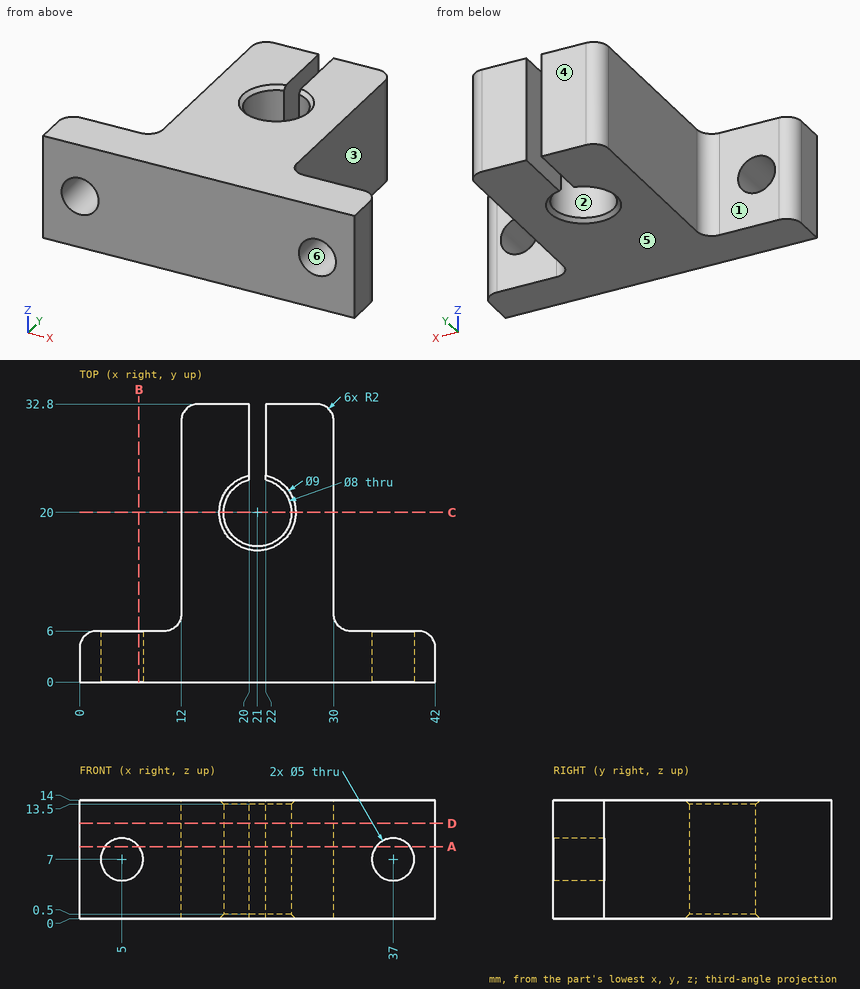
For this review, use the dimensioned drawing (mm, ordinates from the lowest corner) and the shaded views. A direction names the side the tool comes from. Give positions to 0.01 mm unless a question says otherwise; leave off trailing zeros. Loops run counter-clockwise (first coordinate to the right, second up) from the corner with the lowest first, then second, coordinate; pieces in that order, holes last. Notation, with made-up numbers: (22.25, -39) -> (44.25, -39) arc R16 ccw to (44.25, -30) -> close; hole circle Ø6 at (-23, 8.25). An arc over 180 degrees is marked (long way). One line per question, with ' | ' between items. Start each with the question number.
(1) Draft analysis for pull direction Z (two halves, no side actions). For the marked faces 4, 5 and 6, state which applies: +Z half, -Z half, draft (parallel to the pull), parting line (faces both ways), or undercut.
(2) We need section C-C (y = 20). State the section outline as (x, z) points.
(3) For the marked faces 1, 2 and 3, list the 3-axis set-ups (+Z, -Z, +X, -X, +Y, -Y) from which the entire face can be reached by the end or side of a thin tool; tool diameter is ignored.
(4) We need section D-D (z = 11.25). State the section outline as (x, y) points, and give its area (3 significant figures).
(5) Insertion check: P1, Ø2.5, axis at x = 4.5, z = 9, coming from the +Y side; P2, Ø7, axis at y = 27.5, z = 5.5, coming from the -X side; P3, Ø8, axis at x = 7, y = 24.5, coming from the +Z side; P4, Ø1.5, axis at y = 28, z = 12.5, coming from the +X side. Each pin has a flat end and moves straight along its axis. Give the tip position at first contact, or say it passes through.
(6) We need section B-B (x = 7). State the section outline as (y, z) points, and give its area (3 significant figures).
(7) We need section A-A (z = 8.5). State the section outline as (x, y) points.
(8) For line 1 (X direction, y = 25, z = 6.25); line 2 (X direction, y = 20, z = 7.75); line 3 (Z direction, x = 37, y = 2.15), list the stretches that pass through material, from the lowest coordinate up.
The answers:
1) face 4: draft | face 5: -Z half | face 6: undercut
2) outline: (12, 0) -> (16.5, 0) -> (17, 0.5) -> (17, 13.5) -> (16.5, 14) -> (12, 14) -> close; (25, 0.5) -> (25.5, 0) -> (30, 0) -> (30, 14) -> (25.5, 14) -> (25, 13.5) -> close
3) face 1: +Z, -Z, -X, +Y | face 2: +Z, -Z | face 3: +Z, -Z, +X, +Y
4) outline: (0, 0) -> (42, 0) -> (42, 4) arc R2 ccw to (40, 6) -> (32, 6) arc R2 cw to (30, 8) -> (30, 30.8) arc R2 ccw to (28, 32.8) -> (22, 32.8) -> (22, 23.87) arc R4 cw (long way) to (20, 23.87) -> (20, 32.8) -> (14, 32.8) arc R2 ccw to (12, 30.8) -> (12, 8) arc R2 cw to (10, 6) -> (2, 6) arc R2 ccw to (0, 4) -> close | area: 665 mm^2
5) P1: stops at y = 6 | P2: stops at x = 12 | P3: passes through | P4: stops at x = 30
6) outline: (0, 0) -> (6, 0) -> (6, 5.5) -> (0, 5.5) -> close; (0, 8.5) -> (6, 8.5) -> (6, 14) -> (0, 14) -> close | area: 66.0 mm^2
7) outline: (0, 0) -> (3, 0) -> (3, 6) -> (2, 6) arc R2 ccw to (0, 4) -> close; (7, 0) -> (35, 0) -> (35, 6) -> (32, 6) arc R2 cw to (30, 8) -> (30, 30.8) arc R2 ccw to (28, 32.8) -> (22, 32.8) -> (22, 23.87) arc R4 cw (long way) to (20, 23.87) -> (20, 32.8) -> (14, 32.8) arc R2 ccw to (12, 30.8) -> (12, 8) arc R2 cw to (10, 6) -> (7, 6) -> close; (39, 0) -> (42, 0) -> (42, 4) arc R2 ccw to (40, 6) -> (39, 6) -> close
8) line 1: x = 12 to 20, 22 to 30 | line 2: x = 12 to 17, 25 to 30 | line 3: z = 0 to 4.5, 9.5 to 14
